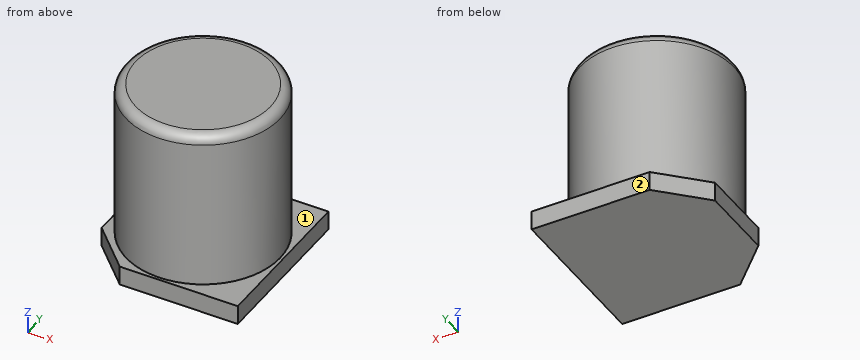
```python
from build123d import *

# Parameters (mm, degrees)
BOSS_EXTRUDE1_DEPTH = 1
SKETCH3_R           = 4
BOSS_EXTRUDE2_DEPTH = 8.3
FILLET2_R           = 0.5


with BuildPart() as part:
    # Sketch2 → Boss-Extrude1 (new body)
    with BuildSketch(Plane.XY):
        Polygon((-1.98, 4.15), (-4.15, 1.98), (-4.15, -1.98), (-1.98, -4.15), (4.15, -4.15), (4.15, 4.15), align=None)
    extrude(amount=BOSS_EXTRUDE1_DEPTH)

    # Sketch3 → Boss-Extrude2 (add)
    with BuildSketch(Plane.XY.offset(1)):
        Circle(SKETCH3_R)
    extrude(amount=BOSS_EXTRUDE2_DEPTH)

    # Fillet2
    fillet2_edges = [part.edges().sort_by_distance(p)[0] for p in [
        (-4, 0, 9.3),
    ]]
    fillet(fillet2_edges, radius=FILLET2_R)


solid = part.part
```
Work out the finished part from the listing and answer in its coordinate system (mm). Face numbers are marked on the shaded views. A direction names the side the tool comes from. Give positions to 0.01 mm unless a question says otherwise; leave off trailing zeros. Write each loop counter-clockwise with the first axis right and the second up, starting at its lowest first coordinate (ties: lowest second). Pieces come first, ordered by that corner, then holes. Notation, with made-up numbers: (56, 89.25) - (106, 89.25) arc R20 ccw to (106, 122.25) - close; hole circle Ø1 at (85, 61). An arc over 180 degrees is marked (long way). Use one line per item in the form item = value.
1. Each of these flat-tipped pins is pushed along its axis until it touches: pin 1 Ø3 at (x, y) = (-1, 0.5) entering from -Z; pin 2 Ø1.5 at (x, z) = (3, 4.5) entering from +Y; pin 3 Ø1 at (y, z) = (-2, 7.5) entering from -X; pin 4 Ø3 at (y, z) = (1.5, 3.5) entering from -X. Where does it stop, or does it pass through?
Filled in:
pin_1 = 0
pin_2 = 3.31
pin_3 = -3.71
pin_4 = -4
2. A cutting plane is placed at A-A (x = 0). Write down the section's boundary in (y, z).
Filled in:
outline = (-4.15, 0) - (4.15, 0) - (4.15, 1) - (4, 1) - (4, 8.8) arc R0.5 ccw to (3.5, 9.3) - (-3.5, 9.3) arc R0.5 ccw to (-4, 8.8) - (-4, 1) - (-4.15, 1) - close
3. For the marked faces 1 and 2, determine the directions among +Z, -Z, +X, -X, +Y, -Y from which every point of the face is accessible in a straight line to the end or side of a thin tool.
Filled in:
face_1 = +Z
face_2 = +Z, -Z, +X, -X, +Y
4. Consider L1, parallel to X at y = -1.75, z = 7; L2, parallel to Y at x = 1.5, z = 3.75; L3, parallel to Z at x = 2.25, y = 3.75. Determine where each line is inside the solid, lowest interval first.
Filled in:
L1 = -3.6 to 3.6
L2 = -3.71 to 3.71
L3 = 0 to 1
5. A cutting plane is placed at C-C (z = 8.5). Write down the section's boundary in (x, y).
Filled in:
outline = circle Ø8 at (0, 0)
